Autodesk Inventor part; units mm, degrees
ref_plane "YZ Plane" through (0, 0, 0) normal (1, 0, 0) x (0, 1, 0)
ref_plane "XZ Plane" through (0, 0, 0) normal (0, 1, 0) x (-1, 0, 0)
ref_plane "XY Plane" through (0, 0, 0) normal (0, 0, 1) x (1, 0, 0)
sketch "Sketch1" plane through (0, 0, 0) normal (0, 1, 0) x (-1, 0, 0)
  line L0 (3.3568, 1.5081) -> (-2.6432, 1.5081)
  line L1 (-2.6432, 1.5081) -> (-2.6432, -4.4919)
  line L2 (-2.6432, -4.4919) -> (3.3568, -4.4919)
  line L3 (3.3568, -4.4919) -> (3.3568, 1.5081)
  point P0 (0, 0)
  dimension "d0" = 6
  dimension "d1" = 6
extrude "Extrusion1" add sketch "Sketch1" along normal blind 3
sketch "Sketch2" plane through (0, 3, 0) normal (0, 1, 0) x (1, 0, 0)
  circle A0 centre (-0.3568, 1.4919) radius 1.5
  line L0 (2.6432, 4.4919) -> (-3.3568, 4.4919)
  line L1 (-3.3568, 4.4919) -> (-3.3568, -1.5081)
  point P0 (0, 0)
  dimension "d4" = 3
  dimension "d5" = 3
  dimension "d6" = 3
extrude "Extrusion2" add sketch "Sketch2" along normal blind 1
sketch "Sketch4" plane through (2.6432, 0, 1.5081) normal (1, 0, 0) x (0, 0, -1)
  line L0 (0, 0) -> (6, 0)
  line L1 (0.5, 0) -> (1.4, 0)
  line L2 (1.4, 0) -> (1.4, 0.7)
  line L3 (1.4, 0.7) -> (0.5, 0.7)
  line L4 (0.5, 0.7) -> (0.5, 0)
  line L5 (0.5, 0) -> (1.4, 0)
  line L6 (1.4, 0) -> (1.4, -3.3)
  line L7 (1.4, -3.3) -> (0.5, -3.3)
  line L8 (0.5, -3.3) -> (0.5, 0)
  line L9 (0, 0) -> (0, 3)
  line L10 (3, 0) -> (3, 3)
  line L11 (0, 3) -> (6, 3)
  line L12 (5.5, 0) -> (4.6, 0)
  line L13 (4.6, 0) -> (4.6, 0.7)
  line L14 (4.6, 0.7) -> (5.5, 0.7)
  line L15 (5.5, 0.7) -> (5.5, 0)
  line L16 (5.5, 0) -> (4.6, 0)
  line L17 (4.6, 0) -> (4.6, -3.3)
  line L18 (4.6, -3.3) -> (5.5, -3.3)
  line L19 (5.5, -3.3) -> (5.5, 0)
  point P0 (1.5081, 0)
  point P1 (1.4, 0.35)
  point P2 (4.4919, 0)
  point P3 (4.6, 0.35)
  dimension "d9" = 0.9
  dimension "d10" = 0.7
  dimension "d11" = 3.3
  dimension "d12" = 0.5
  dimension "d13" = 0
extrude "Extrusion3" add sketch "Sketch4" along normal blind 0.2 contours L13 L14 L15 L0 | L0 L19 L18 L17 | L4 L3 L2 L0 | L0 L6 L7 L8
sketch "Sketch5" plane through (-3.3568, 0, -4.4919) normal (-1, 0, 0) x (0, 0, 1)
  line L0 (0.5, -3.3) -> (0.5, 0.7)
  line L1 (1.4, 0.7) -> (1.4, -3.3)
  line L2 (0.5, 0.7) -> (1.4, 0.7)
  line L3 (1.4, 0.7) -> (1.4, -3.3)
  line L4 (1.4, -3.3) -> (0.5, -3.3)
  line L5 (0.5, -3.3) -> (0.5, 0.7)
  line L6 (5.5, 0.7) -> (5.5, -3.3)
  line L7 (4.6168, 0.7) -> (5.5, 0.7)
  line L8 (5.5, 0.7) -> (5.5, -3.3)
  line L9 (5.5, -3.3) -> (4.6168, -3.3)
  line L10 (4.6168, -3.3) -> (4.6168, 0.7)
  point P0 (4.4919, 0)
extrude "Extrusion4" add sketch "Sketch5" along normal blind 0.2
properties part number "button"
Input: part model. Units: mm. Frame: model coordinates. A direction names the side the tool comes from. Coordinates: 2 decimals unless noted, no trailing zeros. Order: outer loops, then holes, each group sorted by start corner. A loop starts at its lowest first (then second) coordinate and runs counter-clockwise, first axis right, second up. Notation, with made-up numbers: (70.5, 30.5) - (102.5, 30.5) arc R33 cw to (102.5, 67.5) - close; hole circle Ø2 at (69.5, -15). An arc over 180 degrees is marked (long way). Put each result on its own line as item: value.
1. Cut plane B-B on z = -3.7. Return the cut outline in (x, y).
Report:
outline: (-3.56, -3.3) - (-3.36, -3.3) - (-3.36, 0) - (2.64, 0) - (2.64, -3.3) - (2.84, -3.3) - (2.84, 0.7) - (2.64, 0.7) - (2.64, 3) - (-3.36, 3) - (-3.36, 0.7) - (-3.56, 0.7) - close
2. Line query: line 1 along X through (y, z) = (-2.25, -3.75); line 2 along X through (y, z) = (0.75, -4.1); line 3 along Y through (x, z) = (-1.75, -0.6). Output: solid intervals per line, ascending.
Report:
line 1: x = -3.56 to -3.36, 2.64 to 2.84
line 2: x = -3.36 to 2.64
line 3: y = 0 to 3
3. Cut plane C-C on x = 0. Return the cut outline in (y, z), then the cut area to 3 significant figures.
Report:
outline: (0, -4.49) - (3, -4.49) - (3, -2.95) - (4, -2.95) - (4, -0.03) - (3, -0.03) - (3, 1.51) - (0, 1.51) - close
area: 20.9 mm2
4. Cut plane D-D on y = 2.5. Return the cut outline in (x, z), then the cut area to 3 significant figures.
Report:
outline: (-3.36, -4.49) - (2.64, -4.49) - (2.64, 1.51) - (-3.36, 1.51) - close
area: 36.0 mm2
5. Cut plane A-A on y = -1.25. Return the cut outline in (x, z), then the cut area to 3 significant figures.
Report:
outline: (-3.56, -3.99) - (-3.36, -3.99) - (-3.36, -3.09) - (-3.56, -3.09) - close; (-3.56, 0.12) - (-3.36, 0.12) - (-3.36, 1.01) - (-3.56, 1.01) - close; (2.64, -3.99) - (2.84, -3.99) - (2.84, -3.09) - (2.64, -3.09) - close; (2.64, 0.11) - (2.84, 0.11) - (2.84, 1.01) - (2.64, 1.01) - close
area: 0.717 mm2
6. Reachability of faces 4 (the face through (0, 0, -1)), 5 (the face through (-3.557, -1.3, -3.5)), 6 (the face through (-0.552, 3.493, -0.005)) from +Z, -Z, +X, -X, +Y, -Y: full face, straight path, thin tool, end or side. Return the list, or none.
Report:
face 4: +Z, -Z, -Y
face 5: +Z, -Z, -X, +Y, -Y
face 6: +Y
7. Contact query for a flat-ended pin moving along its axis: pin 1 Ø1 at (x, y) = (-0.5, -2) entering from +Z. Output: stop coordinate, or through.
Report:
pin 1: passes through
8. Draft query along Z for faces 1 (the face through (2.643, 1, -1)), 2 (the face through (0, 1, 1.508)), 3 (the face through (0, 4, -2)). Return one class per face: pulls with the +Z half, pulls with the -Z half, needs draft (parallel to the pull), parting line crosses it, or undercut.
Report:
face 1: undercut
face 2: pulls with the +Z half
face 3: needs draft
